Here's how the part is built. I have some questions about the finished solid (model axes, mm). Face numbers are marked on the shaded views. Round coordinates to 2 decimals unless told otherwise and drop trailing zeros. Order: outer loops, then holes, each group sorted by start corner. A loop starts at its lowest first (then second) coordinate and runs counter-clockwise, first axis right, second up. Notation, with made-up numbers: M 5,77 L 9,77 A37 cw 9,115 Z; hole C 18.5,16.5 d3. An arc over 180 degrees is marked long. Answer as CSV lines item,"result". Start each with the question number.
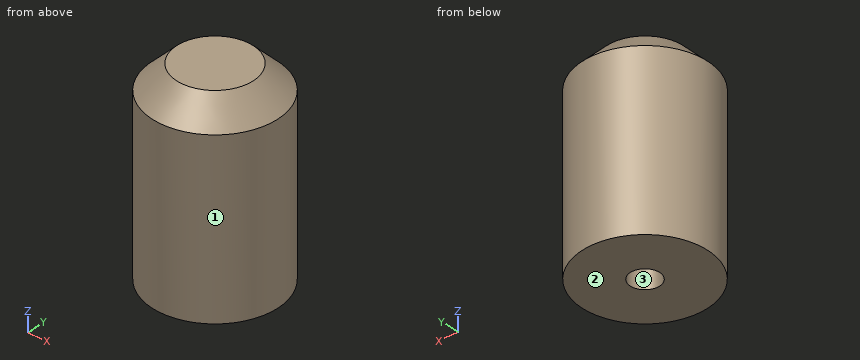
```python
from build123d import *

# Parameters (mm, degrees)
F0_R     = 12.8
F0_R_2   = 3
F1_DEPTH = 40
F2_SIZE  = 5
F3_DEPTH = 10


with BuildPart() as f1:
    # F0 (on Top) → F1 (new body)
    with BuildSketch(Plane.XY):
        Circle(F0_R)
        Circle(F0_R_2, mode=Mode.SUBTRACT)
        Circle(F0_R_2)
    extrude(amount=F1_DEPTH)

    # F2
    f2_edges = [f1.edges().sort_by_distance(p)[0] for p in [
        (-12.8, 0, 40),
    ]]
    chamfer(f2_edges, length=F2_SIZE)

    # F0 (on Top) → F3 (cut)
    with BuildSketch(Plane.XY):
        Circle(F0_R_2)
    extrude(amount=F3_DEPTH, mode=Mode.SUBTRACT)


solid = f1.part
```
Item 1: If I drill on line 1 along Y through (x, z) = (0, 7.25); line 2 along Y through (x, z) = (1, 3.5); line 3 along Y through (x, z) = (3.75, 25.5), over which ranges is the centre line in solid material (lowest first)?
Item 2: If we section it at A-A on x = 0: Please give me the cut outline in (y, z).
Item 3: We'd pull the mould along X, two halves only. Please class the marked faces 1, 2 and 3: pulls with the +X half, pulls with the -X half, needs draft (parallel to the pull), parting line crosses it, or undercut.
Item 4: If we section it at C-C on z = 37: Please give me the cut outline in (x, y).
Item 5: For P1, Ø1.5, axis at x = -10, y = 4, coming from the +Z side; P2, Ø3, axis at x = -4, y = 9.5, coming from the +Z side; P3, Ø8, axis at y = 6, z = 17.5, coming from the -X side, each with a flat end and sliding along its axis, tell me the tip position at first contact or that it passes through.
Item 6: If we section it at D-D on z = 8: Please give me the cut outline in (x, y).
Geometry says:
1,line 1,"-12.8 to -3, 3 to 12.8"
1,line 2,"-12.76 to -2.83, 2.83 to 12.76"
1,line 3,"-12.24 to 12.24"
2,outline,"M -12.8,0 L -3,0 L -3,10 L 3,10 L 3,0 L 12.8,0 L 12.8,35 L 7.8,40 L -7.8,40 L -12.8,35 Z"
3,face 1,"parting line crosses it"
3,face 2,"needs draft"
3,face 3,"undercut"
4,outline,"C 0,0 d21.6"
5,P1,"z = 37.78"
5,P2,"z = 38.99"
5,P3,"x = -12.64"
6,outline,"C 0,0 d25.6; hole C 0,0 d6"
